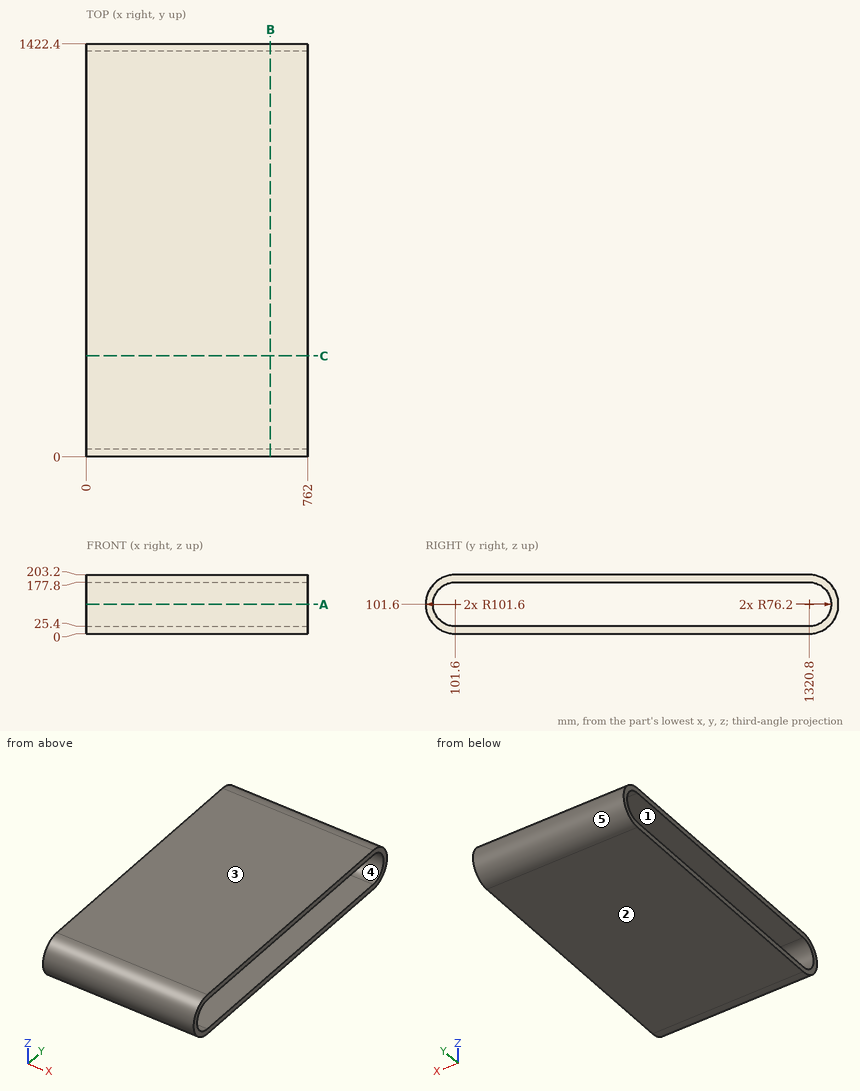
Source: three-view drawing plus pictorial views. Frame: mm from the lowest corner of the part. A direction names the side the tool comes from. Coordinates: 2 decimals unless noted, no trailing zeros. Order: outer loops, then holes, each group sorted by start corner. A loop starts at its lowest first (then second) coordinate and runs counter-clockwise, first axis right, second up. Notation, with made-up numbers: M 36.25,12 L 82.25,12 A24 cw 82.25,37 Z; hole C -27,23 d8. An arc over 180 degrees is marked long. Write each question's results on one line, items separated by ' | '. Start each with the question number.
1. Section A-A, the plane z = 101.6. Return the cut outline in (x, y).
2. Pin query (flat end, axial travel): pin 1 (12 mm diameter, centred on x = 524.5, z = 35.5, fed in from +Y); pin 2 (1.5 mm diameter, centred on x = 668, z = 161, fed in from +Y). Return the tip coordinate at first contact, or that it passes through.
3. Reachability of the marked faces 4 and 5 from +Z, -Z, +X, -X, +Y, -Y: full face, straight path, thin tool, end or side. Return the list, or none.
4. Draft query along Z for the marked faces 1, 2 and 3. Return one class per face: +Z half, -Z half, draft (parallel to the pull), parting line (faces both ways), or undercut.
5. Material intervals for L1, parallel to Z at x = 640, y = 927.5; L2, parallel to Y at x = 227.5, z = 61; L3, parallel to Z at x = 442, y = 93.5, sorted ascending.
6. Section B-B, the plane x = 633.5. Return the cut outline in (y, z).
7. Section C-C, the plane y = 347.5. Return the cut outline in (x, z), then the cut area to 3 significant figures.
Solution:
1) outline: M 0,0 L 762,0 L 762,25.4 L 0,25.4 Z; M 0,1397 L 762,1397 L 762,1422.4 L 0,1422.4 Z
2) pin 1: y = 1402.72 | pin 2: y = 1403.76
3) face 4: +X, -X | face 5: +X, -X, +Y
4) face 1: undercut | face 2: -Z half | face 3: +Z half
5) L1: 0 to 25.4, 177.8 to 203.2 | L2: 8.46 to 37.12, 1385.28 to 1413.94 | L3: 0.32 to 25.83, 177.37 to 202.88
6) outline: M 101.6,0 L 1320.8,0 A101.6 ccw 1320.8,203.2 L 101.6,203.2 A101.6 ccw Z; hole M 101.6,25.4 L 1320.8,25.4 A76.2 ccw 1320.8,177.8 L 101.6,177.8 A76.2 ccw Z
7) outline: M 0,0 L 762,0 L 762,25.4 L 0,25.4 Z; M 0,177.8 L 762,177.8 L 762,203.2 L 0,203.2 Z | area: 38,700 mm²
